from build123d import *

# Parameters (mm, degrees)
BOSS_EXTRUDE1_DEPTH         = 18.25625
CUT_EXTRUDE1_DEPTH          = 590.645135899
F_1_4_CLEARANCE_HOLE1_D     = 7.14248
F_1_4_CLEARANCE_HOLE1_DEPTH = 18.25625


with BuildPart() as part:
    # Sketch1 → Boss-Extrude1 (new body)
    with BuildSketch(Plane(origin=(0, 0, 0), x_dir=(1, 0, 0), z_dir=(0, 1, 0))):
        Polygon((-187.325, -558.8), (187.325, -558.8), (187.325, 0), (66.675, 0), (66.675, -107.95), (-66.675, -107.95), (-66.675, 0), (-187.325, 0), align=None)
    extrude(amount=BOSS_EXTRUDE1_DEPTH)

    # Sketch2 → Cut-Extrude1 (cut, through all)
    with BuildSketch(Plane(origin=(0, 18.25625, 0), x_dir=(1, 0, 0), z_dir=(0, 1, 0))):
        Polygon((-187.325, -201.6125), (-125.4125, -139.7), (-187.325, -77.7875), align=None)
        Polygon((125.4125, -139.7), (187.325, -201.6125), (187.325, -77.7875), align=None)
    extrude(amount=-CUT_EXTRUDE1_DEPTH, mode=Mode.SUBTRACT)

    # 1/4 Clearance Hole1
    with Locations(Plane(origin=(0, 18.25625, 0), x_dir=(1, 0, 0), z_dir=(0, 1, 0))):
        with Locations((-64.29375, -105.56875), (64.29375, -105.56875), (-128.780096045, -139.7), (128.780096045, -139.7)):
            Hole(F_1_4_CLEARANCE_HOLE1_D / 2, depth=F_1_4_CLEARANCE_HOLE1_DEPTH)


solid = part.part
Geometry check sheet. Reference: the model listing, model coordinates, mm. A direction names the side the tool comes from. Coordinates: 2 decimals unless noted, no trailing zeros. Order: outer loops, then holes, each group sorted by start corner. A loop starts at its lowest first (then second) coordinate and runs counter-clockwise, first axis right, second up. Notation, with made-up numbers: (-10, -30.75) - (22, -30.75) arc R18 ccw to (22, -19.75) - close; hole circle Ø7 at (-38, 33). An arc over 180 degrees is marked (long way). One line per item, written item: value.
(1) Sectioned sample at B-B (x = 31). Enter the section's corners in (y, z), and give its area (3 significant figures).
Data:
outline: (0, 107.95) - (18.26, 107.95) - (18.26, 558.8) - (0, 558.8) - close
area: 8,230 mm^2
(2) Release check for a two-part mould opening along Z. For faces 4 (the face through (158.56, 9.26, 106.55)), 5 (the face through (-3, 9, 558.8)), 6 (the face through (-187.325, 9, 378)), 7 (the face through (128, 9, 0)) record: +Z half, -Z half, draft (parallel to the pull), parting line (faces both ways), or undercut.
Data:
face 4: undercut
face 5: +Z half
face 6: draft
face 7: -Z half
(3) Thickness scan on probe 1 along X at (y, z) = (8.5, 101) (1 decimal); probe 2 along Z at (x, y) = (31.5, 11.5); probe 3 along X at (y, z) = (4, 79.5) (1 decimal). Record the ranges inside material, lowest first. Write a range as from..to.
Data:
probe 1: x = -164.1..-66.7, 66.7..164.1
probe 2: z = 107.95..558.8
probe 3: x = -185.6..-66.7, 66.7..185.6
(4) Access from +Z, -Z, +X, -X, +Y, -Y to the whole of each face (thin tool, end or side, straight path). Record for faces 1 (the face through (-157.74, 9.26, 107.37)), 2 (the face through (-66.675, 9, 52)), 3 (the face through (157.74, 9.26, 172.03)).
Data:
face 1: -X, +Y, -Y
face 2: -Z, +Y, -Y
face 3: +X, +Y, -Y
(5) Depth check by flat-ended pin: pin 1 Ø1 at (x, y) = (22.5, 9) entering from -Z; pin 2 Ø2 at (y, z) = (16, 155) entering from +X; pin 3 Ø4 at (y, z) = (14.5, 118) entering from +X. Enter the tip coordinate at first touch or a pass-through.
Data:
pin 1: stops at z = 107.95
pin 2: stops at x = 141.71
pin 3: stops at x = 149.11
